from build123d import *

# Parameters (mm, degrees)
RESSALTO_EXTRUS_O1_START   = -2.81
RESSALTO_EXTRUS_O1_DEPTH   = 2.81
RESSALTO_EXTRUS_O1_START_2 = -11.039175584
RESSALTO_EXTRUS_O1_2_DEPTH = 8.229175584
RESSALTO_EXTRUS_O1_3_DEPTH = 2.81
RESSALTO_EXTRUS_O1_START_3 = -12.229175584
RESSALTO_EXTRUS_O1_4_DEPTH = 1.19
RESSALTO_EXTRUS_O1_START_4 = -10.229175584
RESSALTO_EXTRUS_O1_5_DEPTH = 2
RESSALTO_EXTRUS_O1_6_DEPTH = 11.1
RESSALTO_EXTRUS_O1_7_DEPTH = 13.5
RESSALTO_EXTRUS_O1_START_5 = 11.1
RESSALTO_EXTRUS_O1_8_DEPTH = 2.4
ESBO_O2_R                  = 1.25
CORTE_EXTRUS_O1_DEPTH      = 10
CORTE_EXTRUS_O2_DEPTH      = 11.1
ESBO_O4_W                  = 7.32569207
ESBO_O4_H                  = 2.81
RESSALTO_EXTRUS_O2_DEPTH   = 27
CORTE_EXTRUS_O3_DEPTH      = 10
CORTE_EXTRUS_O3_DEPTH_BACK = 10
ESBO_O5_R                  = 1.7


with BuildPart() as part:
    # Ressalto-extrusão1: read off the stored shape, not the designer's step
    # Ressalto-extrusão1 outline → Ressalto-extrusão1 (new body)
    with BuildSketch(Plane(origin=(0, 12.229175584, 0), x_dir=(1, 0, 0), z_dir=(0, 1, 0)).offset(RESSALTO_EXTRUS_O1_START)):
        Polygon((2.81, -27), (15.31, -27), (15.31, -13.5), (15.31, 0), (2.81, 0), align=None)
        Polygon((4.510961894, -3.75), (4.400461069, -3.513030215), (4.33278837, -3.260472267), (4.31, -3), (4.33278837, -2.739527733), (4.400461069, -2.486969785), (4.510961894, -2.25), (4.660933335, -2.035818585), (4.845818585, -1.850933335), (5.06, -1.700961894), (5.296969785, -1.590461069), (5.549527734, -1.52278837), (5.81, -1.5), (6.070472267, -1.52278837), (6.323030215, -1.590461069), (6.56, -1.700961894), (6.774181415, -1.850933335), (6.959066665, -2.035818585), (7.109038106, -2.25), (7.219538931, -2.486969785), (7.28721163, -2.739527733), (7.31, -3), (7.28721163, -3.260472267), (7.219538931, -3.513030215), (7.109038106, -3.75), (6.959066665, -3.964181415), (6.774181415, -4.149066665), (6.292090707, -4.631157372), (5.327909293, -4.631157372), (4.660933335, -3.964181415), align=None, mode=Mode.SUBTRACT)
    extrude(amount=RESSALTO_EXTRUS_O1_DEPTH)

    # Ressalto-extrus_o1 2 outline → Ressalto-extrus_o1 2 (add)
    with BuildSketch(Plane(origin=(0, 12.229175584, 0), x_dir=(1, 0, 0), z_dir=(0, 1, 0)).offset(RESSALTO_EXTRUS_O1_START_2)):
        Polygon((3.005299462, -7.857883832), (2.81, -7.519615241), (2.81, -11.1), (15.31, -11.1), (15.31, 0), (9.687350269, 0), (11.419401077, -3), (8.614700538, -7.857883832), align=None)
    extrude(amount=RESSALTO_EXTRUS_O1_2_DEPTH)

    # Ressalto-extrus_o1 3 outline → Ressalto-extrus_o1 3 (add)
    with BuildSketch(Plane(origin=(0, 12.229175584, 0), x_dir=(1, 0, 0), z_dir=(0, 1, 0)).offset(RESSALTO_EXTRUS_O1_START_2)):
        Polygon((2.51, -3), (4.242050808, 0), (0, 0), (0, -11.1), (2.81, -11.1), (2.81, -7.519615241), (3.005299462, -7.857883832), (8.614700538, -7.857883832), (11.419401077, -3), (9.687350269, 0), (7.377949192, 0), (9.11, -3), (7.46, -5.857883832), (4.16, -5.857883832), align=None)
    extrude(amount=RESSALTO_EXTRUS_O1_3_DEPTH)

    # Ressalto-extrus_o1 4 outline → Ressalto-extrus_o1 4 (add)
    with BuildSketch(Plane(origin=(0, 12.229175584, 0), x_dir=(1, 0, 0), z_dir=(0, 1, 0)).offset(RESSALTO_EXTRUS_O1_START_3)):
        Polygon((2.51, -3), (4.242050808, 0), (1.932649731, 0), (0.200598923, -3), (3.005299462, -7.857883832), (8.614700538, -7.857883832), (11.419401077, -3), (9.687350269, 0), (7.377949192, 0), (9.11, -3), (7.46, -5.857883832), (4.16, -5.857883832), align=None)
    extrude(amount=RESSALTO_EXTRUS_O1_4_DEPTH)

    # Ressalto-extrus_o1 5 outline → Ressalto-extrus_o1 5 (add)
    with BuildSketch(Plane(origin=(0, 12.229175584, 0), x_dir=(1, 0, 0), z_dir=(0, 1, 0)).offset(RESSALTO_EXTRUS_O1_START_4)):
        Polygon((2.51, -3), (4.16, -5.857883832), (7.46, -5.857883832), (9.11, -3), (7.377949192, 0), (4.242050808, 0), align=None)
        Polygon((4.400461069, -3.513030215), (4.33278837, -3.260472267), (4.31, -3), (4.33278837, -2.739527733), (4.400461069, -2.486969785), (4.510961894, -2.25), (4.660933335, -2.035818585), (4.845818585, -1.850933335), (5.06, -1.700961894), (5.296969785, -1.590461069), (5.549527734, -1.52278837), (5.81, -1.5), (6.070472267, -1.52278837), (6.323030215, -1.590461069), (6.56, -1.700961894), (6.774181415, -1.850933335), (6.959066665, -2.035818585), (7.109038106, -2.25), (7.219538931, -2.486969785), (7.28721163, -2.739527733), (7.31, -3), (7.28721163, -3.260472267), (7.219538931, -3.513030215), (7.109038106, -3.75), (6.959066665, -3.964181415), (6.774181415, -4.149066665), (6.292090707, -4.631157372), (5.327909293, -4.631157372), (4.660933335, -3.964181415), (4.510961894, -3.75), align=None, mode=Mode.SUBTRACT)
    extrude(amount=RESSALTO_EXTRUS_O1_5_DEPTH)

    # Ressalto-extrus_o1 6 outline → Ressalto-extrus_o1 6 (add)
    with BuildSketch(Plane.XY):
        Polygon((17.745732851, 5.751121431), (17.829587792, 6.709587792), (17.745732851, 7.668054154), (17.496715918, 8.597398), (17.090103246, 9.469381688), (16.538249557, 10.257510436), (15.857922643, 10.937837349), (15.31, 11.321496914), (15.31, 2.097678671), (15.857922643, 2.481338236), (16.538249557, 3.161665149), (17.090103246, 3.949793896), (17.496715918, 4.821777584), align=None)
    extrude(amount=RESSALTO_EXTRUS_O1_6_DEPTH)

    # Ressalto-extrus_o1 7 outline → Ressalto-extrus_o1 7 (cut)
    with BuildSketch(Plane.XY):
        Polygon((15.31, 1.19), (15.31, 2.097678671), (15.069793896, 1.929484546), (13.96, 1.19), align=None)
        Polygon((15.264423259, 6.188643259), (15.31, 6.709587792), (15.264423259, 7.230532325), (15.129077862, 7.735648222), (14.908076211, 8.209587792), (14.608133329, 8.637950621), (14.238362829, 9.007721122), (13.81, 9.307664004), (13.33606043, 9.528665655), (12.830944533, 9.664011051), (12.378861267, 9.703563212), (12.368467114, 9.704472583), (12.31, 9.709587792), (12.049527733, 9.686799421), (11.789055467, 9.664011051), (11.536497519, 9.596338353), (11.28393957, 9.528665655), (11.166538463, 9.473920619), (11.049137357, 9.419175584), (2.81, 9.419175584), (2.81, 4), (11.049137357, 4), (11.28393957, 3.89050993), (11.789055467, 3.755164533), (12.31, 3.709587792), (12.830944533, 3.755164533), (13.33606043, 3.89050993), (13.81, 4.111511581), (14.238362829, 4.411454463), (14.608133329, 4.781224963), (14.908076211, 5.209587792), (15.129077862, 5.683527362), align=None)
    extrude(amount=RESSALTO_EXTRUS_O1_7_DEPTH, mode=Mode.SUBTRACT)

    # Ressalto-extrus_o1 8 outline → Ressalto-extrus_o1 8 (cut)
    with BuildSketch(Plane.XY.offset(RESSALTO_EXTRUS_O1_START_5)):
        Polygon((15.31, 9.419175584), (15.31, 9.709587792), (12.378861267, 9.703563212), (12.830944533, 9.664011051), (13.33606043, 9.528665655), (13.570862645, 9.419175584), align=None)
    extrude(amount=RESSALTO_EXTRUS_O1_8_DEPTH, mode=Mode.SUBTRACT)

    # Esboço2 → Corte-extrusão1 (cut)
    with BuildSketch(Plane(origin=(0, 12.229175584, 0), x_dir=(1, 0, 0), z_dir=(0, 1, 0))):
        with Locations(Location((5.81, -13.6, 0), (0, 0, 138.045690322))):
            Circle(ESBO_O2_R)
        with Locations(Location((5.81, -23, 0), (0, 0, 180))):
            Circle(ESBO_O2_R)
    extrude(amount=-CORTE_EXTRUS_O1_DEPTH, mode=Mode.SUBTRACT)

    # Esboço3 → Corte-extrusão2 (cut)
    with BuildSketch(Plane(origin=(0, 0, 0), x_dir=(-1, 0, 0), z_dir=(0, 0, -1))):
        Polygon((-15.31, 11.321496914), (-15.28721163, 9.27601462), (-11.049137357, 9.419175584), (-11.049137357, 5.796906152), (1.171598193, 5.796906152), (1.171598193, -2.184845068), (-19.517418651, -2.184845068), (-19.517418651, 11.321496914), align=None)
    extrude(amount=-CORTE_EXTRUS_O2_DEPTH, mode=Mode.SUBTRACT)

    # Esboço4 → Ressalto-extrusão2 (add)
    with BuildSketch(Plane.XY.offset(27)):
        with Locations((14.647153965, 10.824175584)):
            Rectangle(ESBO_O4_W, ESBO_O4_H)
    extrude(amount=-RESSALTO_EXTRUS_O2_DEPTH)

    # Esboço5 → Corte-extrusão3 (cut, two sides: drawn at the far end of the back side and taken through both)
    with BuildSketch(Plane.XZ.offset(-9.419175584).offset(-CORTE_EXTRUS_O3_DEPTH_BACK)):
        with Locations(Location((14.31, 23, 0), (0, 0, 90))):
            Circle(ESBO_O5_R)
        with Locations(Location((14.31, 4, 0), (0, 0, 90))):
            Circle(ESBO_O5_R)
    extrude(amount=CORTE_EXTRUS_O3_DEPTH + CORTE_EXTRUS_O3_DEPTH_BACK, mode=Mode.SUBTRACT)


solid = part.part
Check sheet for the modelled part. Datum: model origin and axes. Units: mm. A direction names the side the tool comes from. Round coordinates to 2 decimals unless told otherwise and drop trailing zeros. Loops run counter-clockwise (first coordinate to the right, second up) from the corner with the lowest first, then second, coordinate; pieces in that order, holes last. Notation, with made-up numbers: (52.5, 22) - (89.5, 22) arc R23 ccw to (89.5, 53) - close; hole circle Ø10 at (66.25, -16). An arc over 180 degrees is marked (long way). Answer as CSV lines item,"result". Start each with the question number.
Item 1: Section check A-A (z = 13.6). Record the boundary of the cut face in (x, y).
Item 2: Set-up check for faces 4 (the flat face through (6, 11, 4.631)), 5 (the flat face through (10, 11, 0)): record each of +Z, -Z, +X, -X, +Y, -Y from which the full face is reachable in a straight line by a thin tool's end or side.
Item 3: Section check B-B (x = 14.31). Record the boundary of the cut face in (y, z).
Item 4: Section check D-D (z = 10.75). Record the boundary of the cut face in (x, y), and give its area (3 significant figures).
Item 5: Release check for a two-part mould opening along X. For faces 1 (the cylindrical face through (6.08, 10.84, 21.78)), 2 (the flat face through (10, 12.229, 13)), 3 (the flat face through (18.31, 11, 14)) record: +X half, -X half, draft (parallel to the pull), parting line (faces both ways), or undercut.
Item 6: Depth check by flat-ended pin: P1, Ø4, axis at x = 9.5, z = 19, coming from the -Y side. Enter the tip coordinate at first touch or a pass-through.
Item 7: Scan lines: line 1 (Z direction, x = 5.81, y = 10.45); line 2 (Z direction, x = 14.25, y = 11.2); line 3 (X direction, y = 10.8, z = 13.6). Record each from-to range of solid material in increasing order. Write a range as [from, to].
Item 8: Section check C-C (z = 23). Record the boundary of the cut face in (x, y).
Report:
1,outline,"(2.81, 9.42) - (4.56, 9.42) - (4.56, 12.23) - (2.81, 12.23) - close; (7.06, 9.42) - (18.31, 9.42) - (18.31, 12.23) - (7.06, 12.23) - close"
2,face 4,"+Y, -Y"
2,face 5,"-Z, +X, -X, +Y, -Y"
3,outline,"(9.31, 0) - (12.23, 0) - (12.23, 2.3) - (9.31, 2.3) - close; (9.31, 5.7) - (12.23, 5.7) - (12.23, 21.3) - (9.42, 21.3) - (9.42, 11.1) - (9.31, 11.1) - close; (9.42, 24.7) - (12.23, 24.7) - (12.23, 27) - (9.42, 27) - close"
4,outline,"(2.81, 9.42) - (13.57, 9.42) - (13.77, 9.33) - (15.29, 9.28) - (15.29, 9.42) - (18.31, 9.42) - (18.31, 12.23) - (2.81, 12.23) - close"
4,area,"43.7 mm2"
5,face 1,"undercut"
5,face 2,"draft"
5,face 3,"+X half"
6,P1,"stops at y = 9.42"
7,line 1,"z = [0, 1.5], [4.63, 12.35], [14.85, 21.75], [24.25, 27]"
7,line 2,"z = [0, 2.3], [5.7, 21.3], [24.7, 27]"
7,line 3,"x = [2.81, 4.56], [7.06, 18.31]"
8,outline,"(2.81, 9.42) - (4.56, 9.42) - (4.56, 12.23) - (2.81, 12.23) - close; (7.06, 9.42) - (12.61, 9.42) - (12.61, 12.23) - (7.06, 12.23) - close; (16.01, 9.42) - (18.31, 9.42) - (18.31, 12.23) - (16.01, 12.23) - close"
